from build123d import *

# Parameters (mm, degrees)
SKETCH_1_W                                 = 250
SKETCH_1_H                                 = 150
EXTRUDE_1_DEPTH                            = 5
SKETCH_2_W                                 = 15
SKETCH_2_H                                 = 22
EXTRUDE_2_DEPTH                            = 5
MIRROR_2_COPY_1_SKETCH_W                   = 15
MIRROR_2_COPY_1_SKETCH_H                   = 22
MIRROR_2_COPY_1_DEPTH                      = 5
SKETCH_7_R                                 = 1.75
CUT_EXTRUDE_1_DEPTH                        = 148.424556977
MIRROR_4_COPY_1_SKETCH_R                   = 1.75
MIRROR_4_COPY_1_DEPTH                      = 148.424556977
FILLET_1_R                                 = 10
SKETCH_12_W                                = 30
SKETCH_12_H                                = 11
EXTRUDE_4_DEPTH                            = 3
SKETCH_13_W                                = 30
SKETCH_13_H                                = 3
EXTRUDE_5_DEPTH                            = 50
CUT_EXTRUDE_4_DEPTH                        = 192.065433818
CUT_EXTRUDE_4_DEPTH_BACK                   = 192.065433818
SKETCH_16_R                                = 1.75
CUT_EXTRUDE_5_DEPTH                        = 182.950542731
CUT_EXTRUDE_6_DEPTH                        = 182.950542731
CUT_EXTRUDE_6_DEPTH_BACK                   = 5
SKETCH_19_W                                = 6
SKETCH_19_H                                = 20
SKETCH_21_W                                = 210
SKETCH_21_H                                = 30
CUT_EXTRUDE_8_DEPTH                        = 5
SKETCH_23_W                                = 50
SKETCH_23_H                                = 30
EXTRUDE_6_DEPTH                            = 5
SKETCH_24_W                                = 25
SKETCH_24_H                                = 50
CUT_EXTRUDE_9_DEPTH                        = 5
SKETCH_25_W                                = 100
SKETCH_25_H                                = 34
CUT_EXTRUDE_10_DEPTH                       = 5
SKETCH_26_W                                = 50
SKETCH_26_H                                = 15
SKETCH_26_W_2                              = 15
SKETCH_26_H_2                              = 35
CUT_EXTRUDE_11_DEPTH                       = 5
SKETCH_27_R                                = 1.75
CUT_EXTRUDE_12_DEPTH                       = 5
SKETCH_29_R                                = 1.75
CUT_EXTRUDE_13_DEPTH                       = 5
MIRROR_12_AT_THE_SECOND_PLANE_COPY_1_SKE_R = 1.75
MIRROR_12_AT_THE_SECOND_PLANE_COPY_1_DEPTH = 5
CUT_EXTRUDE_14_DEPTH                       = 5
MIRROR_13_AT_THE_SECOND_PLANE_COPY_1_DEPTH = 5
SKETCH_33_W                                = 14.233651272
SKETCH_33_H                                = 34
CUT_EXTRUDE_15_DEPTH                       = 5
SKETCH_34_R                                = 1.75
CUT_EXTRUDE_16_DEPTH                       = 10
SKETCH_35_W                                = 30
SKETCH_35_H                                = 11
CUT_EXTRUDE_17_DEPTH                       = 65


with BuildPart() as part:
    # 草图1 → 凸台-拉伸1 (new body)
    with BuildSketch(Plane(origin=(0, 0, 0), x_dir=(1, 0, 0), z_dir=(0, 1, 0))):
        Rectangle(SKETCH_1_W, SKETCH_1_H)
    extrude(amount=EXTRUDE_1_DEPTH)

    # 草图2 → 凸台-拉伸2 (add)
    with BuildSketch(Plane.XY.offset(22)):
        with Locations((-42.5, 16)):
            Rectangle(SKETCH_2_W, SKETCH_2_H)
    extrude_2 = extrude(amount=-EXTRUDE_2_DEPTH)

    # 镜向1: 凸台-拉伸2 across plane
    add(extrude_2.mirror(Plane.XY))

    # 镜向2: 凸台-拉伸2 across plane
    add(extrude_2.mirror(Plane(origin=(0, 0, 0), x_dir=(0, 0, 1), z_dir=(1, 0, 0))))

    # 镜向2 copy 1 sketch → 镜向2 copy 1 (add)
    with BuildSketch(Plane(origin=(0, 0, -22), x_dir=(-1, 0, 0), z_dir=(0, 0, -1))):
        with Locations((-42.5, 16)):
            Rectangle(MIRROR_2_COPY_1_SKETCH_W, MIRROR_2_COPY_1_SKETCH_H)
    extrude(amount=-MIRROR_2_COPY_1_DEPTH)

    # 草图7 → 切除-拉伸1 (cut, symmetric)
    with BuildSketch(Plane(origin=(0, 5, 0), x_dir=(1, 0, 0), z_dir=(0, 1, 0))):
        with Locations(Location((-115, -55, 0), (0, 0, 270))):
            Circle(SKETCH_7_R)
    cut_extrude_1 = extrude(amount=CUT_EXTRUDE_1_DEPTH, both=True, mode=Mode.SUBTRACT)

    # 镜向3: 切除-拉伸1 across plane
    add(cut_extrude_1.mirror(Plane.XY), mode=Mode.SUBTRACT)

    # 镜向4: 切除-拉伸1 across plane
    add(cut_extrude_1.mirror(Plane(origin=(0, 0, 0), x_dir=(0, 0, 1), z_dir=(1, 0, 0))), mode=Mode.SUBTRACT)

    # 镜向4 copy 1 sketch → 镜向4 copy 1 (cut, symmetric)
    with BuildSketch(Plane(origin=(0, 5, 0), x_dir=(-1, 0, 0), z_dir=(0, 1, 0))):
        with Locations(Location((-115, -55, 0), (0, 0, 270))):
            Circle(MIRROR_4_COPY_1_SKETCH_R)
    extrude(amount=MIRROR_4_COPY_1_DEPTH, both=True, mode=Mode.SUBTRACT)

    # 圆角1
    fillet_1_edges = [part.edges().sort_by_distance(p)[0] for p in [
        (-125, 2.5, -75),
        (125, 2.5, -75),
        (125, 2.5, 75),
        (-125, 2.5, 75),
    ]]
    fillet(fillet_1_edges, radius=FILLET_1_R)

    # 草图12 → 凸台-拉伸4 (add)
    with BuildSketch(Plane(origin=(125, 0, 0), x_dir=(0, 0, -1), z_dir=(1, 0, 0))):
        with Locations((0, 10.5)):
            Rectangle(SKETCH_12_W, SKETCH_12_H)
    extrude(amount=-EXTRUDE_4_DEPTH)

    # 草图13 → 凸台-拉伸5 (add)
    with BuildSketch(Plane(origin=(125, 0, 0), x_dir=(0, 0, -1), z_dir=(1, 0, 0))):
        with Locations((0, 14.5)):
            Rectangle(SKETCH_13_W, SKETCH_13_H)
    extrude(amount=EXTRUDE_5_DEPTH)

    # 草图15 → 切除-拉伸4 (cut, two sides: drawn at the far end of the back side and taken through both)
    with BuildSketch(Plane(origin=(0, 16, 0), x_dir=(1, 0, 0), z_dir=(0, 1, 0)).offset(-CUT_EXTRUDE_4_DEPTH_BACK)):
        Polygon((165, 632.289058028), (165, 15), (165, -15), (165, -632.289058028), (1399.578116055, -632.289058028), (1399.578116055, 632.289058028), align=None)
    extrude(amount=CUT_EXTRUDE_4_DEPTH + CUT_EXTRUDE_4_DEPTH_BACK, mode=Mode.SUBTRACT)

    # 草图16 → 切除-拉伸5 (cut, symmetric)
    with BuildSketch(Plane(origin=(0, 16, 0), x_dir=(1, 0, 0), z_dir=(0, 1, 0))):
        with Locations(Location((135, 8, 0), (0, 0, 270))):
            Circle(SKETCH_16_R)
        with Locations(Location((155, 8, 0), (0, 0, 270))):
            Circle(SKETCH_16_R)
    cut_extrude_5 = extrude(amount=CUT_EXTRUDE_5_DEPTH, both=True, mode=Mode.SUBTRACT)

    # 镜向7: 切除-拉伸5 across plane
    add(cut_extrude_5.mirror(Plane.XY), mode=Mode.SUBTRACT)

    # 草图19 → 切除-拉伸6 (cut, two sides: drawn at the far end of the back side and taken through both)
    with BuildSketch(Plane(origin=(0, 16, 0), x_dir=(1, 0, 0), z_dir=(0, 1, 0)).offset(-CUT_EXTRUDE_6_DEPTH_BACK)):
        with Locations((125, 0)):
            Rectangle(SKETCH_19_W, SKETCH_19_H)
    extrude(amount=CUT_EXTRUDE_6_DEPTH + CUT_EXTRUDE_6_DEPTH_BACK, mode=Mode.SUBTRACT)

    # 草图21 → 切除-拉伸8 (cut)
    with BuildSketch(Plane(origin=(0, 5, 0), x_dir=(1, 0, 0), z_dir=(0, 1, 0))):
        with Locations((0, -60)):
            Rectangle(SKETCH_21_W, SKETCH_21_H)
    cut_extrude_8 = extrude(amount=-CUT_EXTRUDE_8_DEPTH, mode=Mode.SUBTRACT)

    # 草图23 → 凸台-拉伸6 (add)
    with BuildSketch(Plane(origin=(0, 5, 0), x_dir=(1, 0, 0), z_dir=(0, 1, 0))):
        with Locations((0, -60)):
            Rectangle(SKETCH_23_W, SKETCH_23_H)
    extrude_6 = extrude(amount=-EXTRUDE_6_DEPTH)

    # 镜向10: 切除-拉伸8, 凸台-拉伸6 across plane
    add(cut_extrude_8.mirror(Plane.XY), mode=Mode.SUBTRACT)
    add(extrude_6.mirror(Plane.XY))

    # 草图24 → 切除-拉伸9 (cut)
    with BuildSketch(Plane(origin=(0, 5, 0), x_dir=(1, 0, 0), z_dir=(0, 1, 0))):
        with Locations((0, 50)):
            Rectangle(SKETCH_24_W, SKETCH_24_H)
    cut_extrude_9 = extrude(amount=-CUT_EXTRUDE_9_DEPTH, mode=Mode.SUBTRACT)

    # 镜向11: 切除-拉伸9 across plane
    add(cut_extrude_9.mirror(Plane.XY), mode=Mode.SUBTRACT)

    # 草图25 → 切除-拉伸10 (cut)
    with BuildSketch(Plane(origin=(0, 5, 0), x_dir=(1, 0, 0), z_dir=(0, 1, 0))):
        with Locations((-75, 0)):
            Rectangle(SKETCH_25_W, SKETCH_25_H)
    extrude(amount=-CUT_EXTRUDE_10_DEPTH, mode=Mode.SUBTRACT)

    # 草图26 → 切除-拉伸11 (cut)
    with BuildSketch(Plane(origin=(0, 5, 0), x_dir=(1, 0, 0), z_dir=(0, 1, 0))):
        with Locations((62.054344838, 0)):
            Rectangle(SKETCH_26_W, SKETCH_26_H)
        with Locations((62.054344838, 0)):
            Rectangle(SKETCH_26_W_2, SKETCH_26_H_2)
    extrude(amount=-CUT_EXTRUDE_11_DEPTH, mode=Mode.SUBTRACT)

    # 草图27 → 切除-拉伸12 (cut)
    with BuildSketch(Plane(origin=(0, 5, 0), x_dir=(1, 0, 0), z_dir=(0, 1, 0))):
        with Locations(Location((0, 0, 0), (0, 0, 270))):
            Circle(SKETCH_27_R)
    extrude(amount=-CUT_EXTRUDE_12_DEPTH, mode=Mode.SUBTRACT)

    # 草图29 → 切除-拉伸13 (cut)
    with BuildSketch(Plane.XY.offset(22)):
        with Locations((-42.5, 24.75)):
            Circle(SKETCH_29_R)
        with Locations((-42.5, 7.25)):
            Circle(SKETCH_29_R)
    cut_extrude_13 = extrude(amount=-CUT_EXTRUDE_13_DEPTH, mode=Mode.SUBTRACT)

    # 镜向12: 切除-拉伸13 across plane
    add(cut_extrude_13.mirror(Plane(origin=(0, 0, 0), x_dir=(0, 0, 1), z_dir=(1, 0, 0))), mode=Mode.SUBTRACT)

    # 镜向12 at the second plane: 切除-拉伸13 across plane
    add(cut_extrude_13.mirror(Plane.XY), mode=Mode.SUBTRACT)

    # 镜向12 at the second plane copy 1 ske → 镜向12 at the second plane copy 1 (cut)
    with BuildSketch(Plane(origin=(0, 0, -22), x_dir=(-1, 0, 0), z_dir=(0, 0, -1))):
        with Locations((-42.5, 24.75)):
            Circle(MIRROR_12_AT_THE_SECOND_PLANE_COPY_1_SKE_R)
        with Locations((-42.5, 7.25)):
            Circle(MIRROR_12_AT_THE_SECOND_PLANE_COPY_1_SKE_R)
    extrude(amount=-MIRROR_12_AT_THE_SECOND_PLANE_COPY_1_DEPTH, mode=Mode.SUBTRACT)

    # 草图32 → 切除-拉伸14 (cut)
    with BuildSketch(Plane(origin=(0, 5, 0), x_dir=(1, 0, 0), z_dir=(0, 1, 0))):
        with BuildLine():
            Line((-48.4, 26.2), (-36.6, 26.2))
            ThreePointArc((-36.6, 26.2), (-35, 24.6), (-36.6, 23))
            Line((-36.6, 23), (-48.4, 23))
            ThreePointArc((-48.4, 23), (-50, 24.6), (-48.4, 26.2))
        make_face()
    cut_extrude_14 = extrude(amount=-CUT_EXTRUDE_14_DEPTH, mode=Mode.SUBTRACT)

    # 镜向13: 切除-拉伸14 across plane
    add(cut_extrude_14.mirror(Plane(origin=(0, 0, 0), x_dir=(0, 0, 1), z_dir=(1, 0, 0))), mode=Mode.SUBTRACT)

    # 镜向13 at the second plane: 切除-拉伸14 across plane
    add(cut_extrude_14.mirror(Plane.XY), mode=Mode.SUBTRACT)

    # 镜向13 at the second plane copy 1 ske → 镜向13 at the second plane copy 1 (cut)
    with BuildSketch(Plane(origin=(0, 5, 0), x_dir=(-1, 0, 0), z_dir=(0, 1, 0))):
        with BuildLine():
            Line((-48.4, 26.2), (-36.6, 26.2))
            ThreePointArc((-36.6, 26.2), (-35, 24.6), (-36.6, 23))
            Line((-36.6, 23), (-48.4, 23))
            ThreePointArc((-48.4, 23), (-50, 24.6), (-48.4, 26.2))
        make_face()
    extrude(amount=-MIRROR_13_AT_THE_SECOND_PLANE_COPY_1_DEPTH, mode=Mode.SUBTRACT)

    # 草图33 → 切除-拉伸15 (cut)
    with BuildSketch(Plane(origin=(0, 5, 0), x_dir=(1, 0, 0), z_dir=(0, 1, 0))):
        with Locations((42.883174364, 0)):
            Rectangle(SKETCH_33_W, SKETCH_33_H)
    extrude(amount=-CUT_EXTRUDE_15_DEPTH, mode=Mode.SUBTRACT)

    # 草图34 → 切除-拉伸16 (cut)
    with BuildSketch(Plane(origin=(0, 5, 0), x_dir=(1, 0, 0), z_dir=(0, 1, 0))):
        with Locations(Location((105, 8, 0), (0, 0, 270))):
            Circle(SKETCH_34_R)
        with Locations(Location((105, -8, 0), (0, 0, 270))):
            Circle(SKETCH_34_R)
    extrude(amount=-CUT_EXTRUDE_16_DEPTH, mode=Mode.SUBTRACT)

    # 草图35 → 切除-拉伸17 (cut)
    with BuildSketch(Plane.ZY.offset(-122)):
        with Locations((0, 10.5)):
            Rectangle(SKETCH_35_W, SKETCH_35_H)
    extrude(amount=-CUT_EXTRUDE_17_DEPTH, mode=Mode.SUBTRACT)


solid = part.part
CAD build for the part. Positions are in the model's coordinates, mm. A direction names the side the tool comes from. Give positions to 0.01 mm unless a question says otherwise; leave off trailing zeros. Order: outer loops, then holes, each group sorted by start corner. A loop starts at its lowest first (then second) coordinate and runs counter-clockwise, first axis right, second up. Notation, with made-up numbers: (60, 47.25) - (83, 47.25) arc R15 cw to (83, 54.25) - close; hole circle Ø6 at (-16, 50). An arc over 180 degrees is marked (long way). Answer in a Markdown table with one row per item.
1. Probe probe 1 along X at (y, z) = (2.25, -8); probe 2 along X at (y, z) = (2.5, -49); probe 3 along Z at (x, y) = (-115, 3.7). List the from-to ranges inside material, lowest first. Write a range as [from, to].
Data:
| item | result |
|---|---|
| probe 1 | x = [-25, 35.77], [50, 54.55], [69.55, 103.25], [106.75, 125] |
| probe 2 | x = [-125, -105], [-25, -12.5], [12.5, 25], [105, 125] |
| probe 3 | z = [-75, -56.75], [-53.25, -17], [17, 53.25], [56.75, 75] |
2. Tool access for faces 4 (the flat face through (-50, 16, 20)), 5 (the flat face through (42, 3, -23)), 6 (the flat face through (-66, 3, -45)), 7 (the flat face through (-35, 16, -20)), 8 (the flat face through (-64.1, 4.6, 17)): list every direction of +Z, -Z, +X, -X, +Y, -Y with a clear straight run to the whole face (end or side of a thin tool).
Data:
| item | result |
|---|---|
| face 4 | +Z, -Z, -X, +Y |
| face 5 | +Y, -Y |
| face 6 | -Z, +Y, -Y |
| face 7 | +Z, -Z, +Y |
| face 8 | -X, +Y, -Y |
3. Saw through at C-C, the plane z = 49. Give the cut face in (x, y), plus the area to 3 significant figures.
Data:
| item | result |
|---|---|
| outline | (-125, 0) - (-105, 0) - (-105, 5) - (-125, 5) - close; (-25, 0) - (-12.5, 0) - (-12.5, 5) - (-25, 5) - close; (12.5, 0) - (25, 0) - (25, 5) - (12.5, 5) - close; (105, 0) - (125, 0) - (125, 5) - (105, 5) - close |
| area | 325 mm² |
4. Pull direction X, two halves, no side cores. Call faces 1 (the flat face through (-66, 3, 45)), 2 (the flat face through (50, 16, -20)), 3 (the flat face through (-19, 3, 75)): pulls with the +X half, pulls with the -X half, needs draft (parallel to the pull), parting line crosses it, or undercut.
Data:
| item | result |
|---|---|
| face 1 | undercut |
| face 2 | pulls with the +X half |
| face 3 | needs draft |
5. Flat gauge pins, fed straight in: pin 1 (4 mm diameter, centred on x = 41.5, y = 3.5, fed in from -Z); pin 2 (4 mm diameter, centred on y = 18, z = 20, fed in from -X); pin 3 (4 mm diameter, centred on y = 2, z = -2.5, fed in from -X). Where does each tip first touch, or does it go through?
Data:
| item | result |
|---|---|
| pin 1 | stops at z = -45 |
| pin 2 | stops at x = -50 |
| pin 3 | stops at x = -25 |
6. Saw through at A-A, the plane z = -14. Give the cut face in (x, y), plus the area to 3 significant figures.
Data:
| item | result |
|---|---|
| outline | (-25, 0) - (35.77, 0) - (35.77, 5) - (-25, 5) - close; (50, 0) - (54.55, 0) - (54.55, 5) - (50, 5) - close; (69.55, 0) - (125, 0) - (125, 5) - (69.55, 5) - close |
| area | 604 mm² |
7. Saw through at B-B, the plane x = 79. Give the cut face in (y, z).
Data:
| item | result |
|---|---|
| outline | (0, -45) - (5, -45) - (5, -7.5) - (0, -7.5) - close; (0, 7.5) - (5, 7.5) - (5, 45) - (0, 45) - close |
8. Saw through at D-D, the plane y = 17.75. Give the cut face in (x, z).
Data:
| item | result |
|---|---|
| outline | (-50, -22) - (-35, -22) - (-35, -17) - (-50, -17) - close; (-50, 17) - (-35, 17) - (-35, 22) - (-50, 22) - close; (35, -22) - (50, -22) - (50, -17) - (35, -17) - close; (35, 17) - (50, 17) - (50, 22) - (35, 22) - close |
